from build123d import *

# Parameters (mm, degrees)
SKETCH_1_R           = 230
EXTRUDE_1_DEPTH      = 8
SKETCH_2_W           = 80
SKETCH_2_H           = 200
CUT_EXTRUDE_1_DEPTH  = 12
SKETCH_3_R           = 2.75
CUT_EXTRUDE_2_DEPTH  = 12
SKETCH_4_R           = 3.15
CUT_EXTRUDE_3_DEPTH  = 12
SKETCH_5_R           = 3.75
SKETCH_5_R_2         = 2.75
CUT_EXTRUDE_4_DEPTH  = 10
FILLET_1_R           = 10
SKETCH_6_W           = 25
SKETCH_6_H           = 25
CUT_EXTRUDE_5_DEPTH  = 10
SKETCH_7_R           = 2.5
CUT_EXTRUDE_6_DEPTH  = 10
SKETCH_8_W           = 25
SKETCH_8_H           = 25
CUT_EXTRUDE_7_DEPTH  = 10
FILLET_3_R           = 3
SKETCH_10_R          = 2
CUT_EXTRUDE_9_DEPTH  = 326.005785815
SKETCH_11_R          = 2
CUT_EXTRUDE_10_DEPTH = 25
FILLET_4_R           = 3


with BuildPart() as part:
    # 草图1 → 凸台-拉伸1 (new body)
    with BuildSketch(Plane(origin=(0, 0, 0), x_dir=(0, 0, -1), z_dir=(1, 0, 0))):
        Circle(SKETCH_1_R)
    extrude(amount=EXTRUDE_1_DEPTH)

    # 草图2 → 切除-拉伸1 (cut)
    with BuildSketch(Plane(origin=(8, 0, 0), x_dir=(0, 0, -1), z_dir=(1, 0, 0))):
        with Locations((-190, 95)):
            Rectangle(SKETCH_2_W, SKETCH_2_H)
        with Locations((190, 95)):
            Rectangle(SKETCH_2_W, SKETCH_2_H)
    extrude(amount=-CUT_EXTRUDE_1_DEPTH, mode=Mode.SUBTRACT)

    # 草图3 → 切除-拉伸2 (cut)
    with BuildSketch(Plane(origin=(8, 0, 0), x_dir=(0, 0, -1), z_dir=(1, 0, 0))):
        with Locations((-130, 150)):
            Circle(SKETCH_3_R)
        with Locations((-130, 30)):
            Circle(SKETCH_3_R)
        with Locations((130, 30)):
            Circle(SKETCH_3_R)
        with Locations((130, 150)):
            Circle(SKETCH_3_R)
        with Locations((-70, 135)):
            Circle(SKETCH_3_R)
        with Locations((-70, 45)):
            Circle(SKETCH_3_R)
        with Locations((70, 135)):
            Circle(SKETCH_3_R)
        with Locations((70, 45)):
            Circle(SKETCH_3_R)
    extrude(amount=-CUT_EXTRUDE_2_DEPTH, mode=Mode.SUBTRACT)

    # 草图4 → 切除-拉伸3 (cut)
    with BuildSketch(Plane(origin=(8, 0, 0), x_dir=(0, 0, -1), z_dir=(1, 0, 0))):
        with Locations((-14.5, -150)):
            Circle(SKETCH_4_R)
        with Locations((14.5, -150)):
            Circle(SKETCH_4_R)
        with Locations((14.5, -194)):
            Circle(SKETCH_4_R)
        with Locations((-14.5, -194)):
            Circle(SKETCH_4_R)
    extrude(amount=-CUT_EXTRUDE_3_DEPTH, mode=Mode.SUBTRACT)

    # 草图5 → 切除-拉伸4 (cut)
    with BuildSketch(Plane(origin=(8, 0, 0), x_dir=(0, 0, -1), z_dir=(1, 0, 0))):
        with Locations((166.813442197, -81.229769803)):
            Circle(SKETCH_5_R)
        with Locations((108.962557326, -150.173769684)):
            Circle(SKETCH_5_R)
        with Locations((-108.962557326, -150.173769684)):
            Circle(SKETCH_5_R)
        with Locations((-166.813442197, -81.229769803)):
            Circle(SKETCH_5_R)
        with Locations((-11.75, 35)):
            Circle(SKETCH_5_R_2)
        with Locations((11.75, 35)):
            Circle(SKETCH_5_R_2)
        with Locations((95.140628046, -148.366348594)):
            Circle(SKETCH_5_R_2)
        with Locations((162.633327063, -67.931682066)):
            Circle(SKETCH_5_R_2)
        with Locations((180.635371477, -83.037190894)):
            Circle(SKETCH_5_R_2)
        with Locations((113.14267246, -163.471857421)):
            Circle(SKETCH_5_R_2)
        with Locations((-180.635371477, -83.037190894)):
            Circle(SKETCH_5_R_2)
        with Locations((-162.633327063, -67.931682066)):
            Circle(SKETCH_5_R_2)
        with Locations((-95.140628046, -148.366348594)):
            Circle(SKETCH_5_R_2)
        with Locations((-113.14267246, -163.471857421)):
            Circle(SKETCH_5_R_2)
        with Locations((11.75, 140)):
            Circle(SKETCH_5_R_2)
        with Locations((-11.75, 140)):
            Circle(SKETCH_5_R_2)
        with Locations((0, 132.5)):
            Circle(SKETCH_5_R)
        with Locations((0, 42.5)):
            Circle(SKETCH_5_R)
    extrude(amount=-CUT_EXTRUDE_4_DEPTH, mode=Mode.SUBTRACT)

    # 圆角1
    fillet_1_edges = [part.edges().sort_by_distance(p)[0] for p in [
        (4, 174.355957742, -150),
        (4, -5, -150),
        (4, -5, -229.945645751),
        (4, 174.355957742, 150),
        (4, -5, 229.945645751),
        (4, -5, 150),
    ]]
    fillet(fillet_1_edges, radius=FILLET_1_R)

    # 草图6 → 切除-拉伸5 (cut)
    with BuildSketch(Plane(origin=(8, 0, 0), x_dir=(0, 0, -1), z_dir=(1, 0, 0))):
        with Locations((-102.5, -57.5)):
            Rectangle(SKETCH_6_W, SKETCH_6_H)
    extrude(amount=-CUT_EXTRUDE_5_DEPTH, mode=Mode.SUBTRACT)

    # 草图7 → 切除-拉伸6 (cut)
    with BuildSketch(Plane(origin=(8, 0, 0), x_dir=(0, 0, -1), z_dir=(1, 0, 0))):
        with Locations((82.5, -10)):
            Circle(SKETCH_7_R)
        with Locations((82.5, -111)):
            Circle(SKETCH_7_R)
        with Locations((-82.5, -10)):
            Circle(SKETCH_7_R)
        with Locations((-82.5, -111)):
            Circle(SKETCH_7_R)
    extrude(amount=-CUT_EXTRUDE_6_DEPTH, mode=Mode.SUBTRACT)

    # 草图8 → 切除-拉伸7 (cut)
    with BuildSketch(Plane(origin=(8, 0, 0), x_dir=(0, 0, -1), z_dir=(1, 0, 0))):
        with Locations((122.5, -62.5)):
            Rectangle(SKETCH_8_W, SKETCH_8_H)
    extrude(amount=-CUT_EXTRUDE_7_DEPTH, mode=Mode.SUBTRACT)

    # 圆角3
    fillet_3_edges = [part.edges().sort_by_distance(p)[0] for p in [
        (4, -75, -110),
        (4, -50, -110),
        (4, -50, -135),
        (4, -75, -135),
    ]]
    fillet(fillet_3_edges, radius=FILLET_3_R)

    # 草图10 → 切除-拉伸9 (cut, through all)
    with BuildSketch(Plane(origin=(8, 0, 0), x_dir=(0, 0, -1), z_dir=(1, 0, 0))):
        with Locations((168.30023639, -146.301163465)):
            Circle(SKETCH_10_R)
        with Locations((146.301163465, -168.30023639)):
            Circle(SKETCH_10_R)
        with Locations(Location((-146.301163465, -168.30023639, 0), (0, 0, 180))):
            Circle(SKETCH_10_R)
        with Locations(Location((-168.30023639, -146.301163465, 0), (0, 0, 180))):
            Circle(SKETCH_10_R)
    extrude(amount=-CUT_EXTRUDE_9_DEPTH, mode=Mode.SUBTRACT)

    # 草图11 → 切除-拉伸10 (cut)
    with BuildSketch(Plane(origin=(8, 0, 0), x_dir=(0, 0, -1), z_dir=(1, 0, 0))):
        with Locations((100, 190)):
            Circle(SKETCH_11_R)
        with Locations((120, 180)):
            Circle(SKETCH_11_R)
        with Locations((-120, 180)):
            Circle(SKETCH_11_R)
        with Locations((-100, 190)):
            Circle(SKETCH_11_R)
    extrude(amount=-CUT_EXTRUDE_10_DEPTH, mode=Mode.SUBTRACT)

    # 圆角4
    fillet_4_edges = [part.edges().sort_by_distance(p)[0] for p in [
        (4, -70, 115),
        (4, -45, 115),
        (4, -45, 90),
        (4, -70, 90),
    ]]
    fillet(fillet_4_edges, radius=FILLET_4_R)


solid = part.part
Read the model definition and answer for the solid it produces. Units are mm, in the model's axes. Give positions to 0.01 mm unless a question says otherwise; leave off trailing zeros. Write each loop counter-clockwise with the first axis right and the second up, starting at its lowest first coordinate (ties: lowest second). Pieces come first, ordered by that corner, then holes. Notation, with made-up numbers: (-23.5, 60) - (5.5, 60) arc R19 ccw to (5.5, 78) - close; hole circle Ø8 at (87, 54). An arc over 180 degrees is marked (long way). Answer in a Markdown table with one row per item. Add a question column.
Item 1: Section C-C, the plane z = -56 is taken. Write down the section's boundary in (x, y), and give its area (3 significant figures).
Item 2: Find the intervals of material crossed by L1, parallel to Y at x = 3, z = -82.5; L2, parallel to Z at x = 5, y = -56.5; L3, parallel to Y at x = 3.5, z = 130, in increasing order.
Item 3: Flat-ended cylindrical pins translate along their axes: P1, Ø4, axis at x = 2, z = 107, coming from the +Y side; P2, Ø3.5, axis at y = 150, z = 130, coming from the -X side; P3, Ø1.5, axis at x = 5.5, y = -87, coming from the -Z side; P4, Ø4, axis at x = 2.5, y = 97, coming from the -Z side. Find the tip coordinate at first contact, or state that the pin passes through.
Item 4: Section A-A, the plane x = 4 is taken. Count the separate pieces of the cut face and the enclosed holes in it, and give its area (3 significant figures).
Item 5: Section B-B, the plane y = 159 is taken. Write down the section's boundary in (x, z).
Recorded:
| question | item | result |
|---|---|---|
| 1 | outline | (0, -223.08) - (8, -223.08) - (8, 223.08) - (0, 223.08) - close |
| 1 | area | 3,570 mm2 |
| 2 | L1 | y = -214.69 to -113.5, -108.5 to -12.5, -7.5 to 214.69 |
| 2 | L2 | z = -222.95 to -135, -110 to 90, 115 to 222.95 |
| 2 | L3 | y = -189.74 to 27.25, 32.75 to 147.25, 152.75 to 189.74 |
| 3 | P1 | stops at y = 204.63 |
| 3 | P2 | passes through |
| 3 | P3 | stops at z = -213.22 |
| 3 | P4 | stops at z = -150 |
| 4 | separate pieces | 1 |
| 4 | enclosed holes | 44 |
| 4 | area | 144,000 mm2 |
| 5 | outline | (0, -150) - (8, -150) - (8, 150) - (0, 150) - close |
